Source: three-view drawing plus pictorial views. Frame: mm from the lowest corner of the part. A direction names the side the tool comes from. Coordinates: 2 decimals unless noted, no trailing zeros. Write each loop counter-clockwise with the first axis right and the second up, starting at its lowest first coordinate (ties: lowest second). Pieces come first, ordered by that corner, then holes. Notation, with made-up numbers: (14, -37) -> (38, -37) arc R33 ccw to (38, 2) -> close; hole circle Ø1 at (-24, 8.5). An arc over 180 degrees is marked (long way). One line per item, written item: value.
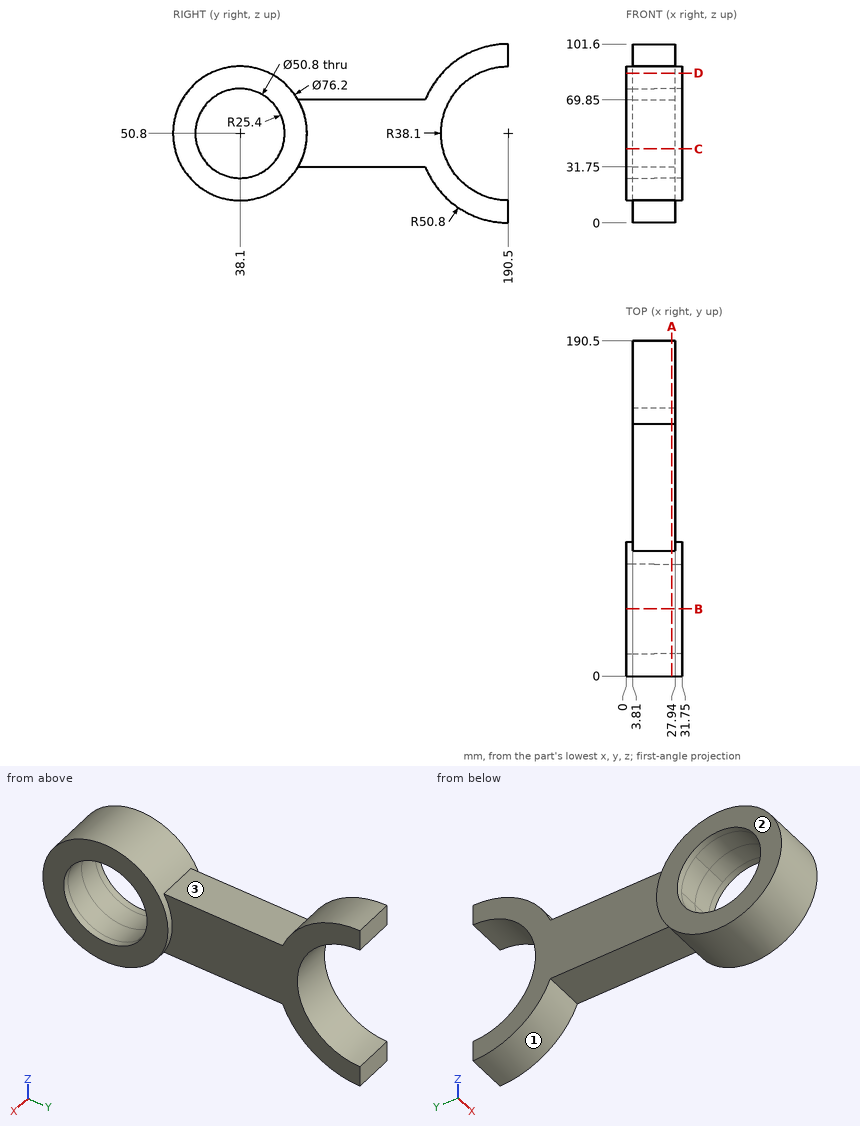
(1) Section B-B (y = 38.1). Return the cut outline in (x, z), then the cut area to 3 significant figures.
Responses:
outline: (0, 12.7) -> (31.75, 12.7) -> (31.75, 25.4) -> (0, 25.4) -> close; (0, 76.2) -> (31.75, 76.2) -> (31.75, 88.9) -> (0, 88.9) -> close
area: 806 mm2
(2) First-contact query: pin 1 (1.5 mm diameter, centred on x = 6.5, z = 77, fed in from +Y); pin 2 (6 mm diameter, centred on x = 27.5, y = 98.5, fed in from -Z); pin 3 (1.5 mm diameter, centred on x = 16, y = 124.5, fed in from +Z). Flat tips, straight axial feed; report the tip coordinate or a pass-through.
Responses:
pin 1: stops at y = 163.57
pin 2: stops at z = 31.75
pin 3: stops at z = 69.85
(3) Section D-D (z = 85). Return the cut outline in (x, y).
Responses:
outline: (0, 21.31) -> (31.75, 21.31) -> (31.75, 54.89) -> (0, 54.89) -> close; (3.81, 152.94) -> (27.94, 152.94) -> (27.94, 173.71) -> (3.81, 173.71) -> close
(4) Line query: line 1 (Z direction, x = 13, y = 38.1); line 2 (Y direction, x = 20, z = 50); line 3 (Z direction, x = 19, y = 171.5). Output: solid intervals per line, ascending. Write a range as [from, to].
Responses:
line 1: z = [12.7, 25.4], [76.2, 88.9]
line 2: y = [0.01, 12.71], [63.49, 152.41]
line 3: z = [3.69, 17.78], [83.82, 97.91]
(5) Section C-C (z = 42). Return the cut outline in (x, y).
Responses:
outline: (0, 1.03) -> (31.75, 1.03) -> (31.75, 14.27) -> (0, 14.27) -> close; (0, 61.93) -> (31.75, 61.93) -> (31.75, 75.17) -> (27.94, 75.17) -> (27.94, 153.43) -> (3.81, 153.43) -> (3.81, 75.17) -> (0, 75.17) -> close
(6) Section A-A (x = 26). Return the cut outline in (y, z).
Responses:
outline: (71.1, 31.75) -> (143.41, 31.75) arc R50.8 ccw to (190.5, 0) -> (190.5, 12.7) arc R38.1 cw to (190.5, 88.9) -> (190.5, 101.6) arc R50.8 ccw to (143.41, 69.85) -> (71.1, 69.85) arc R38.1 ccw (long way) to start; hole circle Ø50.8 at (38.1, 50.8)
(7) Reachability of the marked faces 1, 2 and 3 from +Z, -Z, +X, -X, +Y, -Y: full face, straight path, thin tool, end or side. Return the list, or none.
Responses:
face 1: -Z, +X, -X
face 2: +Z, -Z, -X, +Y, -Y
face 3: +Z, +X, -X
